Geometry check sheet. Reference: the model listing, model coordinates, mm. Face numbers are marked on the shaded views. Give positions to 0.01 mm unless a question says otherwise; leave off trailing zeros. Loops run counter-clockwise (first coordinate to the right, second up) from the corner with the lowest first, then second, coordinate; pieces in that order, holes last.
1. Material ranges on L1, parallel to Z at x = -12.7, y = 1.7; L2, parallel to X at y = 0.35, z = -44.5; L3, parallel to Z at x = 10.5, y = 1.85, recorded low to high.
2. Cross-section at A-A, the plane x = 12.7. Record the cut outline in (y, z).
3. Cross-section at C-C, the plane y = 1.5. Record the cut outline in (x, z) (3 decimals).
4. Cross-section at B-B, the plane z = 69.85. Record the cut outline in (x, y).
5. Go/stop test with a flat-tipped pin: pin 1 Ø3.5 at (x, z) = (34.925, 69.85) entering from +Y. Record where the tip stops, or that it passes through.
6. Cross-section at D-D, the plane z = 44.45. Record the cut outline in (x, y), plus the area to 3 significant figures.
7. Release check for a two-part mould opening along Y. For the marked faces 1 and 2 record: +Y half, -Y half, draft (parallel to the pull), parting line (faces both ways), or undercut.
Autodesk Inventor part; units mm, degrees
ref_plane "Work Plane1" through (-44.45, 0, 69.85) normal (0, 0, 1) x (1, 0, 0)
ref_plane "YZ Plane" through (0, 0, 0) normal (1, 0, 0) x (0, 1, 0)
ref_plane "XZ Plane" through (0, 0, 0) normal (0, 1, 0) x (-1, 0, 0)
sketch "Sketch1" plane through (0, 0, 0) normal (0, 1, 0) x (-1, 0, 0)
  line L0 (44.45, 76.2) -> (-44.45, 76.2)
  line L1 (-44.45, -76.2) -> (44.45, -76.2)
  line L2 (44.45, 76.2) -> (-44.45, -76.2) construction
  line L3 (-44.45, 76.2) -> (44.45, -76.2) construction
  line L4 (0, 0) -> (-53.721, 0) construction
  line L5 (-44.45, 76.2) -> (-44.45, -76.2)
  line L6 (-44.45, -35.3838) -> (-44.45, -76.2)
  line L7 (44.45, 19.05) -> (25.4, 0)
  line L8 (25.4, 0) -> (44.45, -19.05)
  line L9 (44.45, -76.2) -> (44.45, -19.05)
  line L10 (44.45, 19.05) -> (44.45, 76.2)
  point P0 (-12.7, 0)
  point P1 (-44.45, 0)
  dimension "d0" = 88.9
  dimension "d1" = 152.4
  dimension "d4" = 12.7
  dimension "d27" = 90
  dimension "d29" = 19.05
extrude "Extrusion1" add sketch "Sketch1" along normal blind 2.54
ref_plane "Work Plane1" through (-44.45, 0, 69.85) normal (0, 0, 1) x (1, 0, 0)
sketch "Sketch3" plane through (0, 0, 0) normal (0, -1, 0) x (1, 0, 0)
  arc A0 (41.275, 69.85) -> (34.925, 76.2) centre (34.925, 69.85) ccw
  circle A1 centre (34.925, 69.85) radius 2.1844
  circle A2 centre (34.925, -69.85) radius 2.1844
  arc A3 (34.925, -76.2) -> (41.275, -69.85) centre (34.925, -69.85) ccw
  point P0 (0, 0)
  dimension "d22" = 4.3688
  dimension "d23" = 4.3688
extrude "Extrusion3" cut sketch "Sketch3" against normal through all
fillet "Fillet2" radius 3.175 3 edges at (-25.4, 1.27, 0) (-44.45, 1.27, -19.05) (-44.45, 1.27, 19.05)
fillet "Fillet3" radius 3.175 4 edges at (-44.45, 1.27, -76.2) (44.45, 1.27, -76.2) (44.45, 1.27, 76.2) (-44.45, 1.27, 76.2)
sketch "Sketch4" plane through (0, 0, 0) normal (0, -1, 0) x (1, 0, 0)
  circle A0 centre (-12.7, 44.45) radius 2.54
  circle A1 centre (12.7, 44.45) radius 2.54
  circle A2 centre (-12.7, -44.45) radius 2.54
  circle A3 centre (12.7, -44.45) radius 2.54
  line L0 (41.275, -76.2) -> (-41.275, -76.2)
  line L1 (0, -76.2) -> (0, 76.2) construction
  line L2 (-41.275, 76.2) -> (41.275, 76.2)
  line L3 (-12.7, -44.45) -> (-12.7, 44.45) construction
  arc A4 (-27.6451, -2.2451) -> (-27.6451, 2.2451) centre (-29.8901, 0) ccw
  line L4 (-26.7151, 0) -> (44.45, 0) construction
  line L5 (44.45, 73.025) -> (44.45, -73.025)
  point P0 (0, 0)
  dimension "d33" = 25.4
  dimension "d34" = 5.08
  dimension "d35" = 88.9
extrude "Extrusion4" cut sketch "Sketch4" against normal through all
properties part number "match_loader"
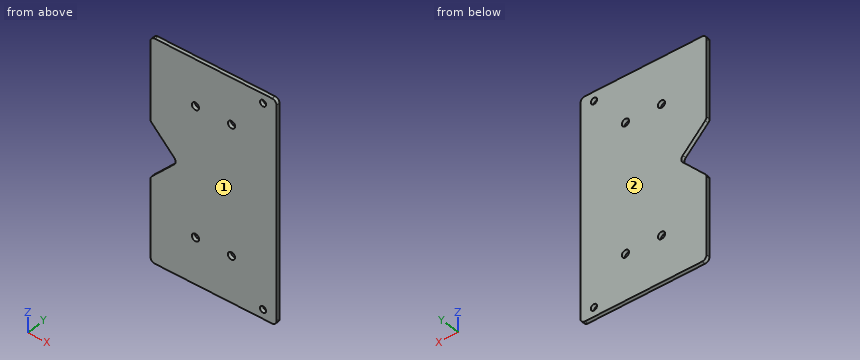
Result:
1. L1: z = -76.2 to -46.99, -41.91 to 41.91, 46.99 to 76.2
1. L2: x = -44.45 to -15.24, -10.16 to 10.16, 15.24 to 44.45
1. L3: z = -76.2 to -45.72, -43.18 to 43.18, 45.72 to 76.2
2. outline: (0, -76.2) - (2.54, -76.2) - (2.54, -46.99) - (0, -46.99) - close; (0, -41.91) - (2.54, -41.91) - (2.54, 41.91) - (0, 41.91) - close; (0, 46.99) - (2.54, 46.99) - (2.54, 76.2) - (0, 76.2) - close
3. outline: (-44.45, -73.025) arc R3.175 ccw to (-41.275, -76.2) - (41.275, -76.2) arc R3.175 ccw to (44.45, -73.025) - (44.45, 73.025) arc R3.175 ccw to (41.275, 76.2) - (-41.275, 76.2) arc R3.175 ccw to (-44.45, 73.025) - (-44.45, 20.365) arc R3.175 ccw to (-43.52, 18.12) - (-27.645, 2.245) arc R3.175 cw to (-27.645, -2.245) - (-43.52, -18.12) arc R3.175 ccw to (-44.45, -20.365) - close; hole circle Ø5.08 at (-12.7, -44.45); hole circle Ø5.08 at (-12.7, 44.45); hole circle Ø5.08 at (12.7, -44.45); hole circle Ø5.08 at (12.7, 44.45); hole circle Ø4.369 at (34.925, -69.85); hole circle Ø4.369 at (34.925, 69.85)
4. outline: (-44.45, 0) - (32.74, 0) - (32.74, 2.54) - (-44.45, 2.54) - close; (37.11, 0) - (44.45, 0) - (44.45, 2.54) - (37.11, 2.54) - close
5. pin 1: passes through
6. outline: (-44.45, 0) - (-15.24, 0) - (-15.24, 2.54) - (-44.45, 2.54) - close; (-10.16, 0) - (10.16, 0) - (10.16, 2.54) - (-10.16, 2.54) - close; (15.24, 0) - (44.45, 0) - (44.45, 2.54) - (15.24, 2.54) - close
6. area: 200 mm2
7. face 1: -Y half
7. face 2: +Y half
